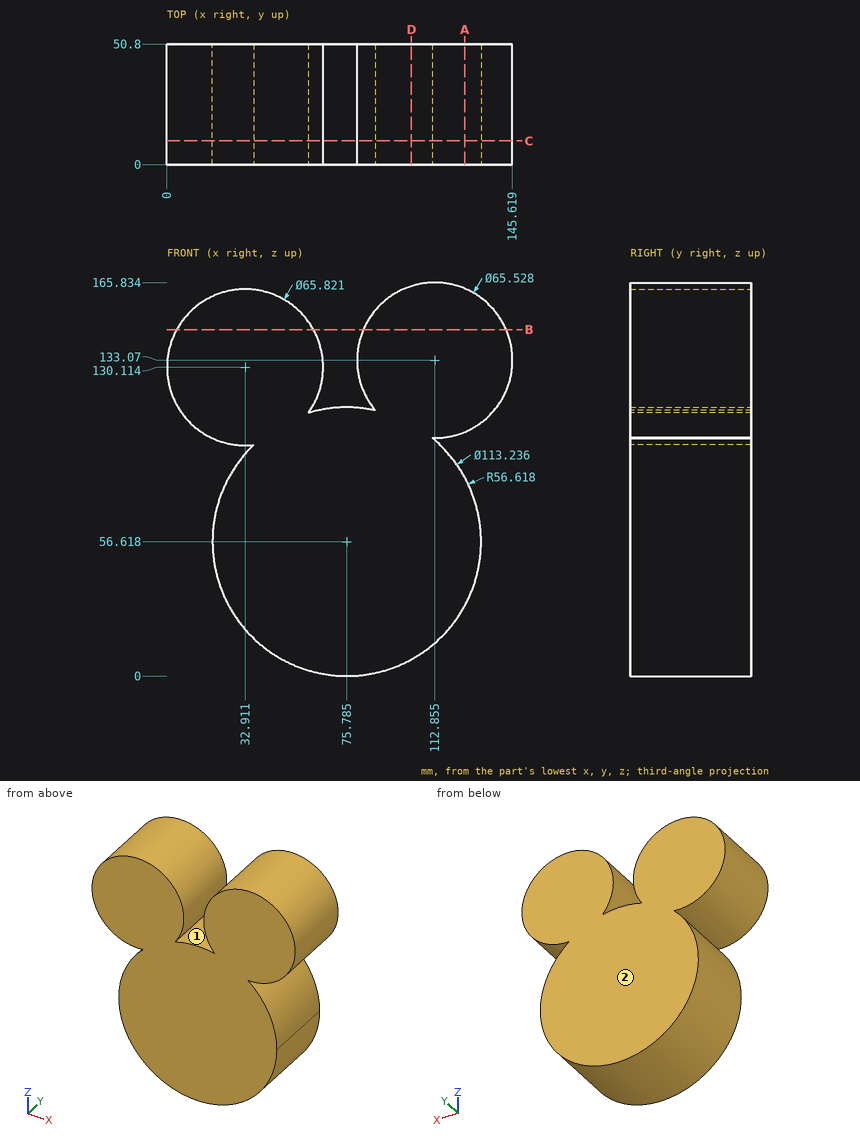
Geometry: see drawing. Coordinates: mm, zero at the bounding-box minimum. Round coordinates to 2 decimals unless told otherwise and drop trailing zeros. Write each loop counter-clockwise with the first axis right and the second up, starting at its lowest first coordinate (ties: lowest second). Pieces come first, ordered by that corner, then holes.
1) Ray query, L1, parallel to Z at x = 123.5, y = 39.5 (1 decimal); L2, parallel to X at y = 6.5, z = 135 (1 decimal); L3, parallel to X at y = 5, z = 151 (1 decimal). Return the intervals inside material, ascending.
2) Cut plane D-D (x = 103). Return the cut outline in (y, z), then the cut area to 3 significant figures.
3) Contact query for flat-ended pins moving along their axis: P1, Ø2, axis at x = 122.5, z = 110.5, coming from the -Y side; P2, Ø4, axis at y = 23.5, z = 39.5, coming from the +X side; P3, Ø4, axis at x = 33, y = 40.5, coming from the -Z side; P4, Ø1, axis at y = 17, z = 82, coming from the +X side. Output: stop coordinate, or through.
4) Draft query along X for the marked faces 1 and 2. Return one class per face: pulls with the +X half, pulls with the -X half, needs draft (parallel to the pull), parting line crosses it, or undercut.
5) Cut plane A-A (x = 125.5). Return the cut outline in (y, z) (1 decimal), then the cut area to 3 significant figures.
6) Cut plane B-B (z = 146). Return the cut outline in (x, y), then the cut area to 3 significant figures.
7) Cut plane C-C (y = 10). Return the cut outline in (x, z) (1 decimal), then the cut area to 3 significant figures.
Geometry says:
1. L1: z = 26.1 to 87.1, 102.1 to 164.1
1. L2: x = 0.4 to 65.5, 80.1 to 145.6
1. L3: x = 7.5 to 58.3, 85.4 to 140.3
2. outline: (0, 6.97) - (50.8, 6.97) - (50.8, 164.32) - (0, 164.32) - close
2. area: 7,990 mm2
3. P1: stops at y = 0
3. P2: stops at x = 130.35
3. P3: stops at z = 17.35
3. P4: stops at x = 126.64
4. face 1: undercut
4. face 2: needs draft
5. outline: (0, 29.5) - (50.8, 29.5) - (50.8, 83.7) - (0, 83.7) - close; (0, 102.8) - (50.8, 102.8) - (50.8, 163.3) - (0, 163.3) - close
5. area: 5,820 mm2
6. outline: (4.09, 0) - (61.73, 0) - (61.73, 50.8) - (4.09, 50.8) - close; (82.75, 0) - (142.96, 0) - (142.96, 50.8) - (82.75, 50.8) - close
6. area: 5,990 mm2
7. outline: (36.5, 97.4) arc R56.6 ccw (long way) to (132.4, 56.6) arc R56.6 ccw to (111.8, 100.3) arc R32.8 ccw (long way) to (87.8, 111.9) arc R56.6 ccw to (59.6, 110.9) arc R32.9 ccw (long way) to start
7. area: 16,700 mm2
